```python
from build123d import *

# Parameters (mm, degrees)
SKETCH1_R           = 1.7
BOSS_EXTRUDE1_DEPTH = 11.3
CUT_EXTRUDE1_REACH  = 28.872
SKETCH2_W           = 6.5
SKETCH2_H           = 6
CHAMFER1_SIZE       = 1.5
CHAMFER1_SIZE2      = 2.400501794
FILLET1_R           = 0.5


with BuildPart() as part:
    # Sketch1 → Boss-Extrude1 (new body)
    with BuildSketch(Plane.XY):
        with BuildLine():
            Line((2.74010383, 9.194695421), (2.74010383, -6.292071669))
            ThreePointArc((2.74010383, -6.292071669), (3.267311624, -7.564863875), (4.54010383, -8.092071669))
            Line((4.54010383, -8.092071669), (4.94010383, -8.092071669))
            ThreePointArc((4.94010383, -8.092071669), (6.212896036, -7.564863875), (6.74010383, -6.292071669))
            Line((6.74010383, -6.292071669), (6.74010383, 9.316577037))
            ThreePointArc((6.74010383, 9.316577037), (6.820858296, 9.879157325), (7.056600411, 10.396306743))
            ThreePointArc((7.056600411, 10.396306743), (7.278226145, 12.999340422), (5.255181103, 14.652274498))
            ThreePointArc((5.255181103, 14.652274498), (4.706198335, 14.850267069), (4.237742883, 15.198308197))
            Line((4.237742883, 15.198308197), (3.085482062, 16.350569018))
            ThreePointArc((3.085482062, 16.350569018), (2.651936559, 16.999415716), (2.499695624, 17.764782581))
            Line((2.499695624, 17.764782581), (2.499695624, 23.862962388))
            ThreePointArc((2.499695624, 23.862962388), (1.125485543, 23.526356004), (-0.200304376, 23.032353678))
            Line((-0.200304376, 23.032353678), (-0.200304376, 14.807928331))
            ThreePointArc((-0.200304376, 14.807928331), (-0.048063441, 14.042561466), (0.385482062, 13.393714769))
            Line((0.385482062, 13.393714769), (1.409315758, 12.369881073))
            ThreePointArc((1.409315758, 12.369881073), (1.757356887, 11.901425621), (1.955349457, 11.352442852))
            ThreePointArc((1.955349457, 11.352442852), (2.120974174, 10.816967431), (2.389933744, 10.325209134))
            ThreePointArc((2.389933744, 10.325209134), (2.650556633, 9.786447131), (2.74010383, 9.194695421))
        make_face()
        with Locations((4.699695624, 11.907928331)):
            Circle(SKETCH1_R, mode=Mode.SUBTRACT)
    extrude(amount=BOSS_EXTRUDE1_DEPTH)

    # Sketch2 → Cut-Extrude1 (cut, up to next)
    with BuildSketch(Plane(origin=(2.499695624, 0, 0), x_dir=(0, 0, -1), z_dir=(1, 0, 0)), mode=Mode.PRIVATE) as cut_extrude1_sk1:
        with Locations((-5.65, 20.862962388)):
            Rectangle(SKETCH2_W, SKETCH2_H)
    cut_extrude1_tool1 = extrude(cut_extrude1_sk1.sketch, amount=-CUT_EXTRUDE1_REACH, mode=Mode.PRIVATE) & part.part
    add(cut_extrude1_tool1.solids().sort_by_distance((2.499696, 20.862962, 5.65))[0], mode=Mode.SUBTRACT)

    # Chamfer1
    chamfer1_edges = [part.edges().sort_by_distance(p)[0] for p in [
        (-0.200304376, 17.862962388, 5.65),
    ]]
    chamfer1_side = [part.faces().sort_by_distance(p)[0] for p in [
        (-0.200304376, 18.920141005, 0.139760929),
    ]]
    chamfer(chamfer1_edges, length=CHAMFER1_SIZE, length2=CHAMFER1_SIZE2, reference=chamfer1_side[0])

    # Fillet1
    fillet1_edges = [part.edges().sort_by_distance(p)[0] for p in [
        (2.499695624, 23.862962388, 10.1),
        (-0.200304376, 23.032353678, 10.1),
        (2.499695624, 23.862962388, 1.2),
        (-0.200304376, 23.032353678, 1.2),
    ]]
    fillet(fillet1_edges, radius=FILLET1_R)


solid = part.part
```
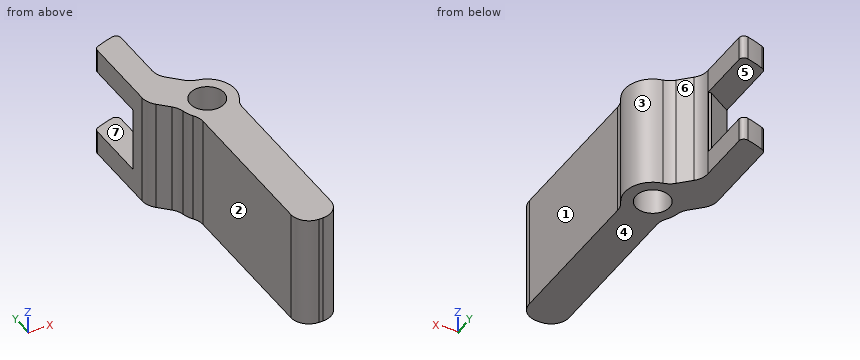
The listing builds one solid part. Answer for the finished solid, in the listing's coordinates (mm). Face numbers are marked on the shaded views. A direction names the side the tool comes from. Round coordinates to 2 decimals unless told otherwise and drop trailing zeros. Loops run counter-clockwise (first coordinate to the right, second up) from the corner with the lowest first, then second, coordinate; pieces in that order, holes last. Notation, with made-up numbers: (-18.75, -12.75) - (19.25, -12.75) arc R27 cw to (19.25, 15.25) - close; hole circle Ø7 at (20, 58). An arc over 180 degrees is marked (long way). Return JSON: item names as keys, results as strings. Group by question number.
1. The part is cut by section C-C on y = 7. Determine the outline of the cut face in (x, z), then the cut area to 3 significant figures.
2. The part is cut by section A-A on x = 6. Determine the outline of the cut face in (y, z), then the cut area to 3 significant figures.
3. Consider probe 1 along X at (y, z) = (5, 4.75); probe 2 along Y at (x, z) = (4.75, 1); probe 3 along Y at (x, z) = (5.5, 1). Determine where each line is inside the solid, lowest interval first.
4. The part is cut by section D-D on z = 1.5. Determine the outline of the cut face in (x, y).
5. The part is cut by section B-B on z = 7.25. Determine the outline of the cut face in (x, y).
6. Each of these flat-tipped pins is pushed along its axis until it touches: P1, Ø1.5, axis at x = 6.5, z = 6, coming from the +Y side; P2, Ø4, axis at x = 2, z = 5.5, coming from the +Y side; P3, Ø3.5, axis at y = 1, z = 4, coming from the +X side. Where does it stop, or does it pass through?
7. The mould has two halves that part along Z. Classify the marked faces 4, 5, 6 and 7: pulls with the +Z half, pulls with the -Z half, needs draft (parallel to the pull), parting line crosses it, or undercut.
8. Which of the six approach directions +Z, -Z, +X, -X, +Y, -Y give full straight-line access (tool end or side, diameter ignored) to the marked faces 1, 2 and 3?
Resolved:
{
 "1": {"outline": "(2.74, 0) - (6.74, 0) - (6.74, 11.3) - (2.74, 11.3) - close", "area": "45.2 mm²"},
 "2": {"outline": "(-7.75, 0) - (10.81, 0) - (10.81, 11.3) - (-7.75, 11.3) - close; (13, 0) - (14.39, 0) - (14.39, 11.3) - (13, 11.3) - close", "area": "225 mm²"},
 "3": {"probe 1": "x = 2.74 to 6.74", "probe 2": "y = -8.09 to 10.21, 13.61 to 14.83", "probe 3": "y = -8 to 10.41, 13.41 to 14.59"},
 "4": {"outline": "(-0.2, 14.81) arc R2 ccw to (0.39, 13.39) - (1.41, 12.37) arc R2 cw to (1.96, 11.35) arc R2.8 ccw to (2.39, 10.33) arc R2 cw to (2.74, 9.19) - (2.74, -6.29) arc R1.8 ccw to (4.54, -8.09) - (4.94, -8.09) arc R1.8 ccw to (6.74, -6.29) - (6.74, 9.32) arc R2 cw to (7.06, 10.4) arc R2.8 ccw to (5.26, 14.65) arc R2 cw to (4.24, 15.2) - (3.09, 16.35) arc R2 cw to (2.5, 17.76) - (2.5, 23.25) arc R0.5 ccw to (1.88, 23.73) arc R12.16 ccw to (0.11, 23.16) arc R0.5 ccw to (-0.2, 22.7) - close; hole circle Ø3.4 at (4.7, 11.91)"},
 "5": {"outline": "(-0.2, 14.81) arc R2 ccw to (0.39, 13.39) - (1.41, 12.37) arc R2 cw to (1.96, 11.35) arc R2.8 ccw to (2.39, 10.33) arc R2 cw to (2.74, 9.19) - (2.74, -6.29) arc R1.8 ccw to (4.54, -8.09) - (4.94, -8.09) arc R1.8 ccw to (6.74, -6.29) - (6.74, 9.32) arc R2 cw to (7.06, 10.4) arc R2.8 ccw to (5.26, 14.65) arc R2 cw to (4.24, 15.2) - (3.09, 16.35) arc R2 cw to (2.5, 17.76) - (2.5, 17.86) - (2.2, 17.86) - (-0.2, 16.36) - close; hole circle Ø3.4 at (4.7, 11.91)"},
 "6": {"P1": "stops at y = 14.5", "P2": "stops at y = 17.86", "P3": "stops at x = 6.74"},
 "7": {"face 4": "pulls with the -Z half", "face 5": "undercut", "face 6": "needs draft", "face 7": "undercut"},
 "8": {"face 1": "+Z, -Z, +X, -Y", "face 2": "+Z, -Z, -X, -Y", "face 3": "+Z, -Z, +X"}
}
